Read the model definition and answer for the solid it produces. Units are mm, in the model's axes. A direction names the side the tool comes from. Give positions to 0.01 mm unless a question says otherwise; leave off trailing zeros. Write each loop counter-clockwise with the first axis right and the second up, starting at its lowest first coordinate (ties: lowest second). Pieces come first, ordered by that corner, then holes. Notation, with made-up numbers: (1.5, 25) - (27.5, 25) arc R17 cw to (27.5, 40) - close; hole circle Ø2 at (-7.75, -18.75). An arc over 180 degrees is marked (long way). Use CSV: the item, a comma, the result in double quotes. Start each with the question number.
from build123d import *

# Parameters (mm, degrees)
SKETCH_1_W          = 300
SKETCH_1_H          = 330
SKETCH_1_R          = 45
EXTRUDE_1_DEPTH     = 6
CUT_EXTRUDE_1_DEPTH = 224.313680727
FILLET_1_R          = 20
SKETCH_3_R          = 9
CUT_EXTRUDE_2_DEPTH = 12


with BuildPart() as part:
    # Эскиз1 → Бобышка-Вытянуть1 (new, symmetric)
    with BuildSketch(Plane.XY):
        Rectangle(SKETCH_1_W, SKETCH_1_H)
        Circle(SKETCH_1_R, mode=Mode.SUBTRACT)
    extrude(amount=EXTRUDE_1_DEPTH, both=True)

    # Эскиз2 → Вырез-Вытянуть1 (cut, through all)
    with BuildSketch(Plane.XY.offset(6)):
        with BuildLine():
            Line((-116.2, 125), (-116.2, 25))
            ThreePointArc((-116.2, 25), (-125, 16.2), (-133.8, 25))
            Line((-133.8, 25), (-133.8, 125))
            ThreePointArc((-133.8, 125), (-125, 133.8), (-116.2, 125))
        make_face()
        with BuildLine():
            Line((-116.2, -125), (-116.2, -25))
            ThreePointArc((-116.2, -25), (-125, -16.2), (-133.8, -25))
            Line((-133.8, -25), (-133.8, -125))
            ThreePointArc((-133.8, -125), (-125, -133.8), (-116.2, -125))
        make_face()
        with BuildLine():
            Line((116.2, -125), (116.2, -25))
            ThreePointArc((116.2, -25), (125, -16.2), (133.8, -25))
            Line((133.8, -25), (133.8, -125))
            ThreePointArc((133.8, -125), (125, -133.8), (116.2, -125))
        make_face()
        with BuildLine():
            Line((116.2, 125), (116.2, 25))
            ThreePointArc((116.2, 25), (125, 16.2), (133.8, 25))
            Line((133.8, 25), (133.8, 125))
            ThreePointArc((133.8, 125), (125, 133.8), (116.2, 125))
        make_face()
    extrude(amount=-CUT_EXTRUDE_1_DEPTH, mode=Mode.SUBTRACT)

    # Скругление1
    fillet_1_edges = [part.edges().sort_by_distance(p)[0] for p in [
        (150, -165, 0),
        (-150, -165, 0),
        (-150, 165, 0),
        (150, 165, 0),
    ]]
    fillet(fillet_1_edges, radius=FILLET_1_R)

    # Эскиз3 → Вырез-Вытянуть2 (cut)
    with BuildSketch(Plane.XY.offset(6)):
        with Locations((-74.599765415, 74.599765415)):
            Circle(SKETCH_3_R)
        with Locations((74.599765415, 74.599765415)):
            Circle(SKETCH_3_R)
        with Locations((74.599765415, -74.599765415)):
            Circle(SKETCH_3_R)
        with Locations((-74.599765415, -74.599765415)):
            Circle(SKETCH_3_R)
    extrude(amount=-CUT_EXTRUDE_2_DEPTH, mode=Mode.SUBTRACT)


solid = part.part
(1) Consider probe 1 along Y at (x, z) = (-73.5, 2.25); probe 2 along X at (y, z) = (88, -0.5); probe 3 along X at (y, z) = (-30.5, 4.5). Determine where each line is inside the solid, lowest interval first.
(2) Given P1, Ø14.5, axis at x = -74.6, y = -74.6, coming from the -Z side; P2, Ø23.5, axis at x = 74.6, y = -74.6, coming from the -Z side, each flat-ended and moving along its own axis, determine where each tip first touches the part or whether it passes through.
(3) The part is cut by section A-A on y = 0. Write down the section's boundary in (x, z), plus the area to 3 significant figures.
(4) For a pull along Y with two mould halves and no side action, classify faces 1 (the face through (125.194, -133.798, 0.084)), 2 (the face through (-2, -165, 0)), 3 (the face through (150, -2, 0)), 4 (the face through (-144.297, 158.986, -0.084)) as pulls with the +Y half, pulls with the -Y half, needs draft (parallel to the pull), parting line crosses it, or undercut.
(5) Which of the six approach directions +Z, -Z, +X, -X, +Y, -Y give full straight-line access (tool end or side, diameter ignored) to faces 5 (the face through (-125.194, -133.798, 0.084)), 6 (the face through (143.986, 159.297, -0.084))?
(6) The part is cut by section D-D on y = 92.5. Write down the section's boundary in (x, z).
(7) The part is cut by section B-B on x = 0. Write down the section's boundary in (y, z), plus the area to 3 significant figures.
(8) The part is cut by section C-C on x = -125. Write down the section's boundary in (y, z).
Reported:
1,probe 1,"-165 to -83.53, -65.67 to 65.67, 83.53 to 165"
1,probe 2,"-150 to -133.8, -116.2 to 116.2, 133.8 to 150"
1,probe 3,"-150 to -133.8, -116.2 to -33.09, 33.09 to 116.2, 133.8 to 150"
2,P1,"through"
2,P2,"z = -6"
3,outline,"(-150, -6) - (-45, -6) - (-45, 6) - (-150, 6) - close; (45, -6) - (150, -6) - (150, 6) - (45, 6) - close"
3,area,"2,520 mm²"
4,face 1,"undercut"
4,face 2,"pulls with the -Y half"
4,face 3,"needs draft"
4,face 4,"pulls with the +Y half"
5,face 5,"+Z, -Z"
5,face 6,"+Z, -Z, +X, +Y"
6,outline,"(-150, -6) - (-133.8, -6) - (-133.8, 6) - (-150, 6) - close; (-116.2, -6) - (116.2, -6) - (116.2, 6) - (-116.2, 6) - close; (133.8, -6) - (150, -6) - (150, 6) - (133.8, 6) - close"
7,outline,"(-165, -6) - (-45, -6) - (-45, 6) - (-165, 6) - close; (45, -6) - (165, -6) - (165, 6) - (45, 6) - close"
7,area,"2,880 mm²"
8,outline,"(-165, -6) - (-133.8, -6) - (-133.8, 6) - (-165, 6) - close; (-16.2, -6) - (16.2, -6) - (16.2, 6) - (-16.2, 6) - close; (133.8, -6) - (165, -6) - (165, 6) - (133.8, 6) - close"
